from build123d import *

# Parameters (mm, degrees)
F0_W     = 3.175
F0_H     = 12.7
F1_DEPTH = 3.175


with BuildPart() as f1:
    # F0 (on Top) → F1 (new body)
    with BuildSketch(Plane.XY):
        Polygon((73.025, 63.5), (73.025, 76.2), (-53.975, 76.2), (-53.975, 63.5), (-57.15, 63.5), (-57.15, 76.2), (-69.85, 76.2), (-69.85, 63.5), (-73.025, 63.5), (-73.025, 50.8), (-69.85, 50.8), (-69.85, 38.1), (-73.025, 38.1), (-73.025, 25.4), (-69.85, 25.4), (-69.85, 12.7), (-73.025, 12.7), (-73.025, 0), (-69.85, 0), (-69.85, -12.7), (-73.025, -12.7), (-73.025, -25.4), (-69.85, -25.4), (-69.85, -38.1), (-73.025, -38.1), (-73.025, -50.8), (-69.85, -50.8), (-69.85, -63.5), (-73.025, -63.5), (-73.025, -76.2), (53.975, -76.2), (53.975, -63.5), (57.15, -63.5), (57.15, -76.2), (69.85, -76.2), (69.85, -63.5), (73.025, -63.5), (73.025, -50.8), (69.85, -50.8), (69.85, -38.1), (73.025, -38.1), (73.025, -25.4), (69.85, -25.4), (69.85, -12.7), (73.025, -12.7), (73.025, 0), (69.85, 0), (69.85, 12.7), (73.025, 12.7), (73.025, 25.4), (69.85, 25.4), (69.85, 38.1), (73.025, 38.1), (73.025, 50.8), (69.85, 50.8), (69.85, 63.5), align=None)
        with Locations((-55.5625, -57.15)):
            Rectangle(F0_W, F0_H, mode=Mode.SUBTRACT)
        with Locations((-55.5625, -31.75)):
            Rectangle(F0_W, F0_H, mode=Mode.SUBTRACT)
        with Locations((-55.5625, -6.35)):
            Rectangle(F0_W, F0_H, mode=Mode.SUBTRACT)
        with Locations((55.5625, -44.45)):
            Rectangle(F0_W, F0_H, mode=Mode.SUBTRACT)
        with Locations((55.5625, -19.05)):
            Rectangle(F0_W, F0_H, mode=Mode.SUBTRACT)
        with Locations((-55.5625, 19.05)):
            Rectangle(F0_W, F0_H, mode=Mode.SUBTRACT)
        with Locations((-55.5625, 44.45)):
            Rectangle(F0_W, F0_H, mode=Mode.SUBTRACT)
        with Locations((55.5625, 6.35)):
            Rectangle(F0_W, F0_H, mode=Mode.SUBTRACT)
        with Locations((55.5625, 31.75)):
            Rectangle(F0_W, F0_H, mode=Mode.SUBTRACT)
        with Locations((55.5625, 57.15)):
            Rectangle(F0_W, F0_H, mode=Mode.SUBTRACT)
    extrude(amount=F1_DEPTH)


solid = f1.part
Input: part model. Units: mm. Frame: model coordinates. A direction names the side the tool comes from. Round coordinates to 2 decimals unless told otherwise and drop trailing zeros. Loops run counter-clockwise (first coordinate to the right, second up) from the corner with the lowest first, then second, coordinate; pieces in that order, holes last. Notation, with made-up numbers: (39, 10.25) -> (81, 10.25) arc R23 cw to (81, 25.25) -> close; hole circle Ø8 at (51.5, 77). An arc over 180 degrees is marked (long way). Answer as a JSON object with one key per item and string values. Group by question number.
1) Reachability of faces 1 (the flat face through (-71, -63.5, 2)), 2 (the flat face through (69.85, 57, 2)), 3 (the flat face through (-56, 50.8, 2)), 4 (the flat face through (-69.85, 70, 2)) from +Z, -Z, +X, -X, +Y, -Y: full face, straight path, thin tool, end or side. Return the list, or none.
2) Pin query (flat end, axial travel): pin 1 (1.6 mm diameter, centred on y = 71, z = 1.5, fed in from -X); pin 2 (1.6 mm diameter, centred on y = -17, z = 2.5, fed in from +X); pin 3 (1.6 mm diameter, centred on x = 71.5, z = 1.5, fed in from -Y). Return the tip coordinate at first contact, or that it passes through.
3) Section query B-B on z = 0.6. State how many separate pieces and enclosed holes the cut face has, plus the area to 3 significant figures.
4) Ray query, L1, parallel to Y at x = 55, z = 2.4; L2, parallel to X at y = 3, z = 3 (3 decimals); L3, parallel to X at y = 47, z = 2.25 (3 decimals). Return the intervals inside material, ascending.
5) Draft query along X for faces 5 (the flat face through (71, 0, 2)), 6 (the flat face through (-57.15, 44, 2)), 7 (the flat face through (53.975, 57, 2)), 8 (the flat face through (-69.85, -6, 2)). Return one class per face: +X half, -X half, draft (parallel to the pull), parting line (faces both ways), or undercut.
6) Section query A-A on y = 31. Output: boundary loops of the cut face in (x, z) (3 decimals).
Reply:
{
 "1": {"face 1": "+Z, -Z, -X", "face 2": "+Z, -Z, +X", "face 3": "+Z, -Z", "face 4": "+Z, -Z, -X, +Y"},
 "2": {"pin 1": "stops at x = -69.85", "pin 2": "stops at x = 69.85", "pin 3": "stops at y = -63.5"},
 "3": {"separate pieces": "1", "enclosed holes": "10", "area": "21,300 mm2"},
 "4": {"L1": "y = -63.5 to -50.8, -38.1 to -25.4, -12.7 to 0, 12.7 to 25.4, 38.1 to 50.8, 63.5 to 76.2", "L2": "x = -73.025 to 53.975, 57.15 to 69.85", "L3": "x = -69.85 to -57.15, -53.975 to 73.025"},
 "5": {"face 5": "draft", "face 6": "undercut", "face 7": "undercut", "face 8": "-X half"},
 "6": {"outline": "(-73.025, 0) -> (53.975, 0) -> (53.975, 3.175) -> (-73.025, 3.175) -> close; (57.15, 0) -> (69.85, 0) -> (69.85, 3.175) -> (57.15, 3.175) -> close"}
}
